from build123d import *

# Parameters (mm, degrees)
SKETCH1_W           = 120
SKETCH1_H           = 80
BOSS_EXTRUDE1_DEPTH = 50
SHELL1_T            = -2
SKETCH3_R           = 2.5
SKETCH3_W           = 37.6
SKETCH3_H           = 19
SKETCH3_W_2         = 10
SKETCH3_H_2         = 20
SKETCH3_W_3         = 20
SKETCH3_H_3         = 10
CUT_EXTRUDE1_DEPTH  = 2
SKETCH4_R           = 3.5
SKETCH4_W           = 20
SKETCH4_H           = 5
CUT_EXTRUDE2_DEPTH  = 2
SKETCH5_W           = 118
SKETCH5_H           = 78
CUT_EXTRUDE3_DEPTH  = 4
CUT_EXTRUDE3_TAPER  = 1
SKETCH6_W           = 11.841510552
SKETCH6_H           = 5
SKETCH6_W_2         = 20
SKETCH6_H_2         = 5.927680675
CUT_EXTRUDE4_DEPTH  = 4


with BuildPart() as part:
    # Sketch1 → Boss-Extrude1 (new body)
    with BuildSketch(Plane(origin=(0, 0, 0), x_dir=(1, 0, 0), z_dir=(0, 1, 0))):
        Rectangle(SKETCH1_W, SKETCH1_H)
    extrude(amount=BOSS_EXTRUDE1_DEPTH)

    # Shell1
    shell1_openings = [part.faces().sort_by_distance(p)[0] for p in [
        (0, 50, 0),
    ]]
    offset(amount=SHELL1_T, openings=shell1_openings, kind=Kind.INTERSECTION)

    # Sketch3 → Cut-Extrude1 (cut)
    with BuildSketch(Plane.XZ):
        with Locations((-50, 31.648007145)):
            Circle(SKETCH3_R)
        with Locations((-50, 23.107977616)):
            Circle(SKETCH3_R)
        with Locations((0, 23.513536142)):
            Rectangle(SKETCH3_W, SKETCH3_H)
        with Locations((-50, -25)):
            Rectangle(SKETCH3_W_2, SKETCH3_H_2)
        with Locations((20, -30)):
            Rectangle(SKETCH3_W_3, SKETCH3_H_3)
        with Locations((-20, -30)):
            Rectangle(SKETCH3_W_3, SKETCH3_H_3)
        with Locations((50, -25)):
            Rectangle(SKETCH3_W_2, SKETCH3_H_2)
    extrude(amount=-CUT_EXTRUDE1_DEPTH, mode=Mode.SUBTRACT)

    # Sketch4 → Cut-Extrude2 (cut)
    with BuildSketch(Plane.ZY.offset(60)):
        with Locations((5, 10)):
            Circle(SKETCH4_R)
        with Locations((-25, 6.740257278)):
            Rectangle(SKETCH4_W, SKETCH4_H)
    extrude(amount=-CUT_EXTRUDE2_DEPTH, mode=Mode.SUBTRACT)

    # Sketch5 → Cut-Extrude3 (cut)
    with BuildSketch(Plane(origin=(0, 50, 0), x_dir=(1, 0, 0), z_dir=(0, 1, 0))):
        Rectangle(SKETCH5_W, SKETCH5_H)
    extrude(amount=-CUT_EXTRUDE3_DEPTH, taper=CUT_EXTRUDE3_TAPER, mode=Mode.SUBTRACT)

    # Sketch6 → Cut-Extrude4 (cut)
    with BuildSketch(Plane(origin=(60, 0, 0), x_dir=(0, 0, -1), z_dir=(1, 0, 0))):
        with Locations((-4.084800513, 8.280260813)):
            Rectangle(SKETCH6_W, SKETCH6_H)
        with Locations((-4.084800513, 16.026907298)):
            Rectangle(SKETCH6_W, SKETCH6_H)
        with Locations((25, 7.816420476)):
            Rectangle(SKETCH6_W_2, SKETCH6_H_2)
    extrude(amount=-CUT_EXTRUDE4_DEPTH, mode=Mode.SUBTRACT)


solid = part.part
Geometry: final body of the model. Coordinates: model frame, mm. A direction names the side the tool comes from. Round coordinates to 2 decimals unless told otherwise and drop trailing zeros. Loops run counter-clockwise (first coordinate to the right, second up) from the corner with the lowest first, then second, coordinate; pieces in that order, holes last. Notation, with made-up numbers: (69.25, -4) - (100.25, -4) arc R23 ccw to (100.25, 7) - close; hole circle Ø9 at (-2.5, 81). An arc over 180 degrees is marked (long way). Write each question's results on one line, items separated by ' | '. Start each with the question number.
1) Cut plane A-A on y = 44.5. Return loops of the section in (x, z).
2) Mould query, pull axis X, two halves, no side actions, for faces 4 (the face through (-47.615, 0.986, 32.399)), 5 (the face through (60, 25, 1)), 6 (the face through (-1, 25, -40)). Classes: released by +X, released by -X, zero draft, split by the parting line, or undercut.
3) Cut plane B-B on y = 17. Return loops of the section in (x, z), then the cut area to 3 significant figures.
4) Line query: probe 1 along Z at (x, y) = (-50, 1); probe 2 along Z at (x, y) = (-25, 4); probe 3 along X at (y, z) = (42, 29). Output: solid intervals per line, ascending. Write a range as [from, to].
5) Access query for faces 1 (the face through (-1, 0, -1)), 2 (the face through (-1, 24, 38)), 3 (the face through (-59.014, 6.895, 6.615)). Directions: +Z, -Z, +X, -X, +Y, -Y. A direction counts if a zero-diameter tool reaches every point of the face in a straight line with its end or side. Return the directions, or none.
6) First-contact query: P1, Ø1.5, axis at x = -45, z = 26.5, coming from the +Y side. Flat tip, straight axial feed; report the tip coordinate or a pass-through.
7) Cut plane C-C on x = 15.5. Count the separate pieces of the cut face and the enclosed holes in it, then the cut area to 3 significant figures.
Verdict:
1) outline: (-60, -40) - (60, -40) - (60, 40) - (-60, 40) - close; hole (-58, -38) - (58, -38) - (58, 38) - (-58, 38) - close
2) face 4: undercut | face 5: released by +X | face 6: zero draft
3) outline: (-60, -40) - (60, -40) - (60, -1.84) - (58, -1.84) - (58, -38) - (-58, -38) - (-58, 38) - (58, 38) - (58, 10.01) - (60, 10.01) - (60, 40) - (-60, 40) - close | area: 760 mm2
4) probe 1: z = [-40, -35], [-15, 20.61], [25.61, 29.15], [34.15, 40] | probe 2: z = [-40, -38], [38, 40] | probe 3: x = [-60, -58], [58, 60]
5) face 1: +Z, -Z, +X, -X, -Y | face 2: +Y | face 3: -X
6) P1: stops at y = 2
7) separate pieces: 3 | enclosed holes: 0 | area: 286 mm2
